For this review, take the finished solid that the model builds, in its own axes (mm). Face numbers are marked on the shaded views. A direction names the side the tool comes from. Coordinates: 2 decimals unless noted, no trailing zeros. Write each loop counter-clockwise with the first axis right and the second up, starting at its lowest first coordinate (ties: lowest second). Pieces come first, ordered by that corner, then holes.
```python
from build123d import *

# Parameters (mm, degrees)
F0_W     = 1828.8
F0_H     = 762
F1_DEPTH = 304.8
F2_T     = -2.54
F4_D     = 76.2
F4_DEPTH = 12.7
F5_W     = 12.7
F5_H     = 756.92
F6_DEPTH = 304.8


with BuildPart() as f1:
    # F0 (on Front) → F1 (new body)
    with BuildSketch(Plane.XZ):
        with Locations((453.363994, 8.726588)):
            Rectangle(F0_W, F0_H)
    extrude(amount=F1_DEPTH)

    # F2
    f2_openings = [f1.faces().sort_by_distance(p)[0] for p in [
        (453.363994, 0, 8.726588),
    ]]
    offset(amount=F2_T, openings=f2_openings)

    # F4
    with Locations(Plane(origin=(0, 0, -372.273412), x_dir=(1, 0, 0), z_dir=(0, 0, -1))):
        with Locations((-236.677806, 152.4), (-84.277806, 152.4), (389.872461, 152.4), (542.272461, 152.4), (991.005794, 152.4), (1143.405794, 152.4)):
            Hole(F4_D / 2, depth=F4_DEPTH)

    # F5 (on face) → F6 (join)
    with BuildSketch(Plane(origin=(0, -302.26, 0), x_dir=(-1, 0, 0), z_dir=(0, 1, 0))):
        with Locations((-760.289127, 8.726588)):
            Rectangle(F5_W, F5_H)
        with Locations((-146.455794, 8.726588)):
            Rectangle(F5_W, F5_H)
    extrude(amount=F6_DEPTH)


solid = f1.part
```
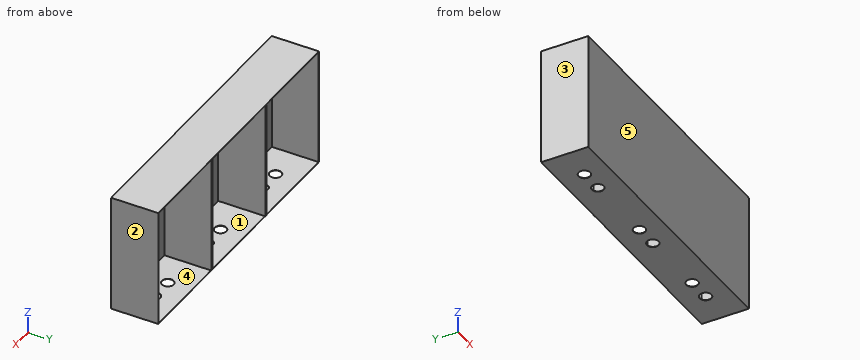
1) Consider section C-C (x = 169). Give the boundary of the cut face in (y, z).
2) Clearance check with flat-ended pins moving along their axes: P1, Ø12, axis at x = 301, z = -226, coming from the +Y side; P2, Ø0.8, axis at x = 761.5, y = 0.5, coming from the -Z side. State where each tip first meets the part, or that it passes through.
3) Consider section A-A (y = -266.5). Give the boundary of the cut face in (x, z), then the cut area to 3 significant figures.
4) The part is to be moulded in two halves that separate along X. For the marked faces 3, 4 and 5, say which applies: pulls with the +X half, pulls with the -X half, needs draft (parallel to the pull), parting line crosses it, or undercut.
5) Consider section B-B (z = -266). Give the boundary of the cut face in (x, y).
6) Tool access review of the marked faces 1 and 2: name each direction out of +Z, -Z, +X, -X, +Y, -Y from which nothing blocks a thin tool from reaching the whole face with its end or side.
7) For L1, parallel to X at y = -190.5, z = -239; L2, parallel to Z at x = -383, y = -243; L3, parallel to Y at x = 337, z = 322.5, list the stretches that pass through material, from the lowest coordinate up.
8) Consider section D-D (x = 377). Give the boundary of the cut face in (y, z).
Results:
1. outline: (-304.8, -372.27) - (0, -372.27) - (0, -369.73) - (-302.26, -369.73) - (-302.26, 387.19) - (0, 387.19) - (0, 389.73) - (-304.8, 389.73) - close
2. P1: stops at y = -302.26
2. P2: stops at z = -369.73
3. outline: (-461.04, -372.27) - (1367.76, -372.27) - (1367.76, 389.73) - (-461.04, 389.73) - close; hole (-458.5, -369.73) - (140.11, -369.73) - (140.11, 387.19) - (-458.5, 387.19) - close; hole (152.81, -369.73) - (753.94, -369.73) - (753.94, 387.19) - (152.81, 387.19) - close; hole (766.64, -369.73) - (1365.22, -369.73) - (1365.22, 387.19) - (766.64, 387.19) - close
3. area: 32,400 mm2
4. face 3: pulls with the -X half
4. face 4: undercut
4. face 5: needs draft
5. outline: (-461.04, -304.8) - (1367.76, -304.8) - (1367.76, 0) - (1365.22, 0) - (1365.22, -302.26) - (766.64, -302.26) - (766.64, 2.54) - (753.94, 2.54) - (753.94, -302.26) - (152.81, -302.26) - (152.81, 2.54) - (140.11, 2.54) - (140.11, -302.26) - (-458.5, -302.26) - (-458.5, 0) - (-461.04, 0) - close
6. face 1: +Y
6. face 2: +Z, -Z, +X, +Y, -Y
7. L1: x = -461.04 to -458.5, 140.11 to 152.81, 753.94 to 766.64, 1365.22 to 1367.76
7. L2: z = -372.27 to -369.73, 387.19 to 389.73
7. L3: y = -304.8 to -302.26
8. outline: (-304.8, -372.27) - (-188.26, -372.27) - (-188.26, -369.73) - (-302.26, -369.73) - (-302.26, 387.19) - (0, 387.19) - (0, 389.73) - (-304.8, 389.73) - close; (-116.54, -372.27) - (0, -372.27) - (0, -369.73) - (-116.54, -369.73) - close
